Input: part model. Units: mm. Frame: model coordinates. A direction names the side the tool comes from. Round coordinates to 2 decimals unless told otherwise and drop trailing zeros. Answer as CSV lines item,"result". Start each with the question number.
1) Line query: L1, parallel to X at y = 2, z = 1; L2, parallel to X at y = 2.25, z = 1.25; L3, parallel to Z at x = -7.25, y = -8.5. Output: solid intervals per line, ascending.
2) Access query for faces 1 (the face through (-6.5, -8.9, -3)), 2 (the face through (-1, -11, 3)), 3 (the face through (1.11, -11.04, 0.08)), 4 (the face through (-1.09, -11.01, 5.92)), 5 (the face through (6.7, 9.34, -1.48)). Directions: +Z, -Z, +X, -X, +Y, -Y. A direction counts if a zero-diameter tool reaches every point of the face in a straight line with its end or side. Return the directions, or none.
3) Section query A-A, the plane z = 1. State how many separate pieces and enclosed holes the cut face has, and give its area (3 significant figures).
4) First-contact query: P1, Ø3, axis at y = -4.5, z = 3.5, coming from the -X side; P2, Ø4, axis at x = -3.5, z = 3.5, coming from the +Y side; P3, Ø0.6, axis at x = 0, z = 2.5, coming from the -Y side. Flat tips, straight axial feed; report the tip coordinate or a pass-through.
5) Mould query, pull axis X, two halves, no side actions, for faces 6 (the face through (-6.5, 8.9, -3)), 7 (the face through (3.13, 4.55, 2.96)). Classes: +X half, -X half, draft (parallel to the pull), parting line (faces both ways), or undercut.
```python
from build123d import *

# Parameters (mm, degrees)
SKETCH_R      = 0.5
PAD_DEPTH     = 6
FILLET_R      = 0.25
FILLET001_R   = 0.25
SKETCH001_R   = 0.5
SKETCH001_R_2 = 2.5
PAD001_DEPTH  = 3


with BuildPart() as part:
    # Sketch → Pad (new body)
    with BuildSketch(Plane.XY):
        with BuildLine():
            ThreePointArc((1.75, -12.124356), (0, 12.25), (-1.75, -12.124356))
            Line((-1.75, -12.124356), (-0.5, -10.25))
            Line((-0.5, -10.25), (0.5, -10.25))
            Line((0.5, -10.25), (1.75, -12.124356))
        make_face()
        with Locations((-3.526712, -4.854102)):
            Circle(SKETCH_R, mode=Mode.SUBTRACT)
        with Locations((-5.706339, -1.854102)):
            Circle(SKETCH_R, mode=Mode.SUBTRACT)
        with Locations((-5.706339, 1.854102)):
            Circle(SKETCH_R, mode=Mode.SUBTRACT)
        with Locations((-3.526712, 4.854102)):
            Circle(SKETCH_R, mode=Mode.SUBTRACT)
        with Locations((0, 6)):
            Circle(SKETCH_R, mode=Mode.SUBTRACT)
        with Locations((3.526712, 4.854102)):
            Circle(SKETCH_R, mode=Mode.SUBTRACT)
        with Locations((5.706339, 1.854102)):
            Circle(SKETCH_R, mode=Mode.SUBTRACT)
        with Locations((5.706339, -1.854102)):
            Circle(SKETCH_R, mode=Mode.SUBTRACT)
        with Locations((3.526712, -4.854102)):
            Circle(SKETCH_R, mode=Mode.SUBTRACT)
    extrude(amount=PAD_DEPTH)

    # Fillet
    fillet_edges = [part.edges().sort_by_distance(p)[0] for p in [
        (0, 12.25, 6),
        (1.125, -11.187178, 6),
        (0, -10.25, 6),
        (-1.125, -11.187178, 6),
        (0, 12.25, 0),
        (-1.125, -11.187178, 0),
        (0, -10.25, 0),
        (1.125, -11.187178, 0),
    ]]
    fillet(fillet_edges, radius=FILLET_R)

    # Fillet001
    fillet001_edges = [part.edges().sort_by_distance(p)[0] for p in [
        (-1.75, -12.124356, 3),
        (-0.5, -10.25, 3),
        (0.5, -10.25, 3),
        (1.75, -12.124356, 3),
    ]]
    fillet(fillet001_edges, radius=FILLET001_R)

    # Sketch001 (on Face8 of Fillet001) → Pad001 (join)
    with BuildSketch(Plane(origin=(0, 0, 0), x_dir=(1, 0, 0), z_dir=(0, 0, -1))):
        with Locations((-6.465638, 8.899187)):
            Circle(SKETCH001_R)
        with Locations((-10.461622, 3.399187)):
            Circle(SKETCH001_R)
        with Locations((-10.461622, -3.399187)):
            Circle(SKETCH001_R)
        with Locations((-6.465638, -8.899187)):
            Circle(SKETCH001_R)
        with Locations((0, -11)):
            Circle(SKETCH001_R)
        with Locations((6.465638, -8.899187)):
            Circle(SKETCH001_R)
        with Locations((10.461622, -3.399187)):
            Circle(SKETCH001_R)
        with Locations((10.461622, 3.399187)):
            Circle(SKETCH001_R)
        with Locations((6.465638, 8.899187)):
            Circle(SKETCH001_R)
        Circle(SKETCH001_R_2)
    extrude(amount=PAD001_DEPTH)


solid = part.part
```
Findings:
1,L1,"x = -12.09 to -6.18, -5.23 to 5.23, 6.18 to 12.09"
1,L2,"x = -12.04 to -6.01, -5.4 to 5.4, 6.01 to 12.04"
1,L3,"z = 0 to 6"
2,face 1,"-Z, +X, -X, +Y, -Y"
2,face 2,"+Z, -Z, -Y"
2,face 3,"-Z, -Y"
2,face 4,"+Z, -Y"
2,face 5,"-Z"
3,separate pieces,"1"
3,enclosed holes,"9"
3,area,"460 mm^2"
4,P1,"stops at x = -11.88"
4,P2,"stops at y = 12.16"
4,P3,"stops at y = -10.25"
5,face 6,"draft"
5,face 7,"undercut"
